Can you work these out from the model? Positions are in its coordinate system, mm. A direction names the side the tool comes from. Round coordinates to 2 decimals unless told otherwise and drop trailing zeros. Write each loop counter-clockwise with the first axis right and the second up, starting at its lowest first coordinate (ties: lowest second). Pieces come first, ordered by that corner, then holes.
Q1. If we section it at D-D (y = 12): Please give me the cut outline in (x, z), plus the area to 3 significant figures.
Q2. I'm going to push flat-ended pins straight in: pin 1 Ø21 at (x, y) = (36.5, 13) entering from -Z; pin 2 Ø3 at (x, y) = (67.5, 135.5) entering from -Z. Where does each tip first touch, or does it pass through?
Q3. Please list where these lines run through material, in increasing order: line 1 along X through (y, z) = (117.5, 26); line 2 along Y through (x, z) = (17, 27); line 3 along Z through (x, y) = (75, 63.5).
Q4. For faces 1 (the flat face through (44, 12, 30)), 2 (the flat face through (44, 135, 25)), 3 (the flat face through (55, 107, 23)), 4 (the flat face through (53.24, 118, 26)), which set-ups out of +Z, -Z, +X, -X, +Y, -Y let a thin tool reach every point of the face, with its end or its side?
Q5. If we section it at B-B (x = 42): Please give me the cut outline in (y, z), plus the area to 3 significant figures.
Q6. If we section it at A-A (z = 23.5): Please give me the cut outline in (x, y), plus the area to 3 significant figures.
Q7. We'd pull the mould along X, two halves only. Please class faces 5 (the flat face through (0, 80, 29)), 6 (the flat face through (46.76, 118, 26)), 7 (the flat face through (44, 66, 35)): +X half, -X half, draft (parallel to the pull), parting line (faces both ways), or undercut.
Q8. If we section it at C-C (y = 113): Please give me the cut outline in (x, z), plus the area to 3 significant figures.
from build123d import *

# Parameters (mm, degrees)
EXTRUDE_DEPTH     = 40
BOX004_W          = 10
BOX004_H          = 33
BOX004_DEPTH      = 11
BOX004_ROLL_ANGLE = 10
BOX_W             = 90
BOX_H             = 23
BOX_DEPTH         = 30
BOX002_W          = 90
BOX002_H          = 110
BOX002_DEPTH      = 10
BOX003_W          = 90
BOX003_H          = 110
BOX003_DEPTH      = 5
BOX003_ROLL_ANGLE = 11
BOX001_W          = 90
BOX001_H          = 35
BOX001_DEPTH      = 35
CHAMFER_SIZE      = 5
FILLET_R          = 5
FILLET001_R       = 5
FILLET002_R       = 1
CHAMFER001_SIZE   = 2


with BuildPart() as extrude_body:
    # Sketch → Extrude (new body)
    with BuildSketch(Plane.XY):
        with BuildLine():
            ThreePointArc((3.239725, 4.799999), (0, 8.039724), (-3.239725, 4.799999))
            Line((-3.239725, 4.799999), (-3.239725, -15.2))
            ThreePointArc((-3.239725, -15.2), (0, -18.439725), (3.239725, -15.2))
            Line((3.239725, 4.799999), (3.239725, -15.2))
        make_face()
    extrude(amount=EXTRUDE_DEPTH)


with BuildPart() as extrude_body_1:
    # Extrude placement: moved
    add(extrude_body.part.moved(Location((50, 123, 0))))


with BuildPart() as cubo:
    # Box004 → Box004 (new body)
    with BuildSketch(Plane.XY):
        with Locations((5, 16.5)):
            Rectangle(BOX004_W, BOX004_H)
    extrude(amount=BOX004_DEPTH)


with BuildPart() as cubo_1:
    # Box004 roll: moved
    add(cubo.part.rotate(Axis((0, 0, 0), (1, 0, 0)), BOX004_ROLL_ANGLE))


with BuildPart() as cubo_2:
    # Box004 placement: moved
    add(cubo_1.part.moved(Location((45, 100.726682, 17.263939))))


with BuildPart() as obj1:
    # Box → Box (new body)
    with BuildSketch(Plane.XY):
        with Locations((45, 11.5)):
            Rectangle(BOX_W, BOX_H)
    extrude(amount=BOX_DEPTH)


with BuildPart() as soporte_superior:
    # Box002 → Box002 (new body)
    with BuildSketch(Plane(origin=(0, 27, 25), x_dir=(1, 0, 0), z_dir=(0, 0, 1))):
        with Locations((45, 55)):
            Rectangle(BOX002_W, BOX002_H)
    extrude(amount=BOX002_DEPTH)


with BuildPart() as soporte_superior001:
    # Box003 → Box003 (new body)
    with BuildSketch(Plane.XY):
        with Locations((45, 55)):
            Rectangle(BOX003_W, BOX003_H)
    extrude(amount=BOX003_DEPTH)


with BuildPart() as soporte_superior001_1:
    # Box003 roll: moved
    add(soporte_superior001.part.rotate(Axis((0, 0, 0), (1, 0, 0)), BOX003_ROLL_ANGLE))


with BuildPart() as soporte_superior001_2:
    # Box003 placement: moved
    add(soporte_superior001_1.part.moved(Location((0, 25.96455, 0.597369))))


with BuildPart() as obj2:
    # Box001 → Box001 (new body)
    with BuildSketch(Plane(origin=(0, -6, 0), x_dir=(1, 0, 0), z_dir=(0, 0, 1))):
        with Locations((45, 17.5)):
            Rectangle(BOX001_W, BOX001_H)
    extrude(amount=BOX001_DEPTH)

    # Fusion: union soporte superior, soporte superior001
    add(soporte_superior.part)
    add(soporte_superior001_2.part)

    # Cut: cut obj1
    add(obj1.part, mode=Mode.SUBTRACT)

    # Chamfer
    chamfer_edges = [obj2.edges().sort_by_distance(p)[0] for p in [
        (45, 29, 25),
        (45, 29, 6.280985),
    ]]
    chamfer(chamfer_edges, length=CHAMFER_SIZE)

    # Fillet
    fillet_edges = [obj2.edges().sort_by_distance(p)[0] for p in [
        (45, -6, 35),
    ]]
    fillet(fillet_edges, radius=FILLET_R)

    # Fillet001
    fillet001_edges = [obj2.edges().sort_by_distance(p)[0] for p in [
        (45, 137, 35),
    ]]
    fillet(fillet001_edges, radius=FILLET001_R)

    # Fillet002
    fillet002_edges = [obj2.edges().sort_by_distance(p)[0] for p in [
        (45, -6, 0),
        (45, 0, 0),
        (45, 29, 0),
        (45, 23, 0),
    ]]
    fillet(fillet002_edges, radius=FILLET002_R)

    # Chamfer001
    chamfer001_edges = [obj2.edges().sort_by_distance(p)[0] for p in [
        (45, 0, 30),
        (45, 23, 30),
    ]]
    chamfer(chamfer001_edges, length=CHAMFER001_SIZE)

    # Fusion001: union Cubo
    add(cubo_2.part)

    # Cut001: cut Extrude body
    add(extrude_body_1.part, mode=Mode.SUBTRACT)


solid = obj2.part
A:
1. outline: (0, 30) - (90, 30) - (90, 35) - (0, 35) - close
1. area: 450 mm2
2. pin 1: stops at z = 0.13
2. pin 2: stops at z = 25
3. line 1: x = 0 to 46.76, 53.24 to 90
3. line 2: y = -6 to 0, 23 to 137
3. line 3: z = 7.89 to 12.99, 25 to 35
4. face 1: -Z, +X, -X
4. face 2: +X, -X, +Y
4. face 3: +X
4. face 4: +Z, -Z
5. outline: (-6, 1) arc R1 ccw to (-5, 0) - (-1, 0) arc R1 ccw to (0, 1) - (0, 28) - (2, 30) - (21, 30) - (23, 28) - (23, 1) arc R1 ccw to (24, 0) - (28, 0) arc R1 ccw to (29, 1) - (29, 1.19) - (133.94, 21.59) - (133.28, 25) - (137, 25) - (137, 30) arc R5 ccw to (132, 35) - (-1, 35) arc R5 ccw to (-6, 30) - close; hole (29, 11.28) - (33.91, 7.24) - (125.3, 25) - (34, 25) - (29, 20) - close
5. area: 2,160 mm2
6. outline: (0, -6) - (90, -6) - (90, 0) - (0, 0) - close; (0, 23) - (90, 23) - (90, 32.5) - (0, 32.5) - close; (0, 117.58) - (45, 117.58) - (45, 99.63) - (55, 99.63) - (55, 117.58) - (90, 117.58) - (90, 133.57) - (0, 133.57) - close; hole (46.76, 107.8) arc R3.24 ccw to (53.24, 107.8) - (53.24, 127.8) arc R3.24 ccw to (46.76, 127.8) - close
6. area: 2,850 mm2
7. face 5: -X half
7. face 6: undercut
7. face 7: draft
8. outline: (0, 17.52) - (46.76, 17.52) - (46.76, 35) - (0, 35) - (0, 25) - (45, 25) - (45, 22.61) - (0, 22.61) - close; (53.24, 17.52) - (90, 17.52) - (90, 22.61) - (55, 22.61) - (55, 25) - (90, 25) - (90, 35) - (53.24, 35) - close
8. area: 1,270 mm2
